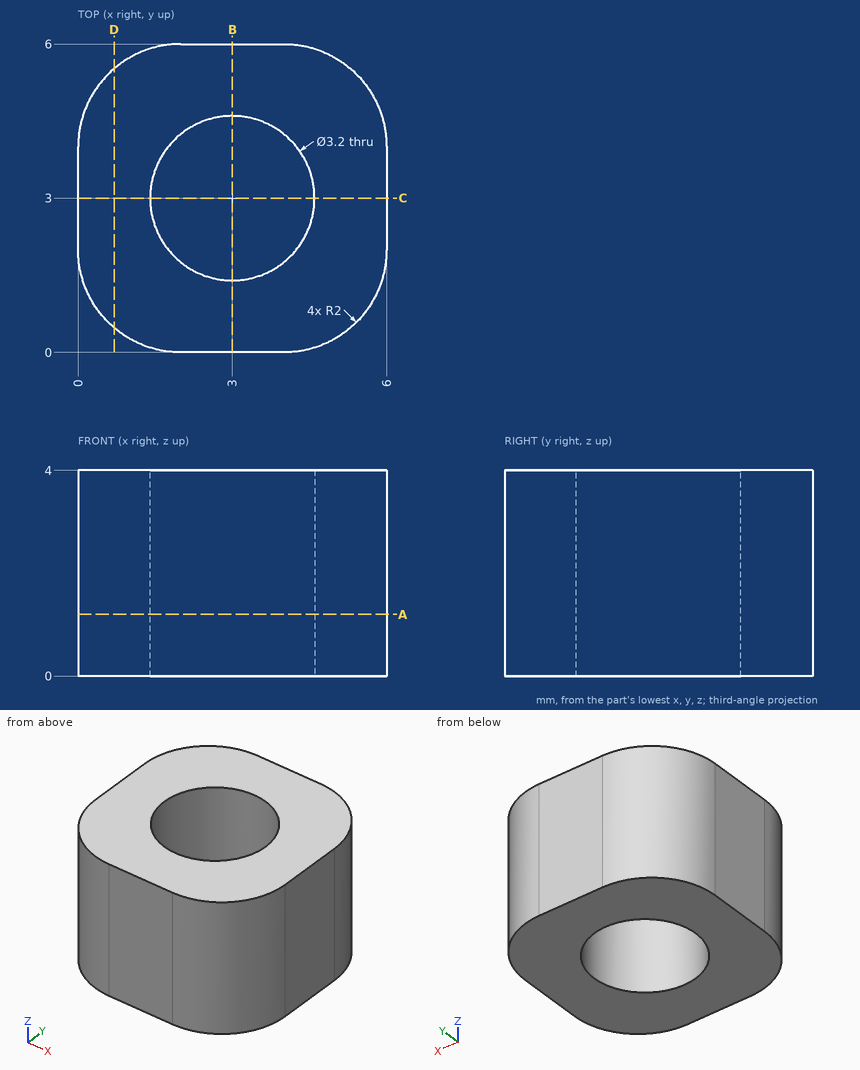
Check sheet for the drawn part. Datum: minimum x, y, z corner. Units: mm. Give positions to 0.01 mm unless a question says otherwise; leave off trailing zeros. Write each loop counter-clockwise with the first axis right and the second up, starting at its lowest first coordinate (ties: lowest second). Pieces come first, ordered by that corner, then holes. Notation, with made-up numbers: M 40.5,-5 L 74.5,-5 A17 cw 74.5,24 Z; hole C 0,-35.75 d10. An arc over 180 degrees is marked long. Write item = value, one per line.
(1) Go/stop test with flat-tipped pins: pin 1 Ø1.5 at (x, z) = (1, 0.5) entering from +Y; pin 2 Ø2 at (y, z) = (5, 2) entering from -X. Record where each tip stops, or that it passes through.
Found:
pin_1 = 5.98
pin_2 = 0
(2) Material ranges on line 1 (Y direction, x = 3, z = 3.1); line 2 (Y direction, x = 3.5, z = 3.65), recorded low to high.
Found:
line_1 = 0 to 1.4, 4.6 to 6
line_2 = 0 to 1.48, 4.52 to 6
(3) Sectioned sample at D-D (x = 0.7). Record the cut outline in (y, z), then the cut area to 3 significant figures.
Found:
outline = M 0.48,0 L 5.52,0 L 5.52,4 L 0.48,4 Z
area = 20.2 mm2
(4) Sectioned sample at B-B (x = 3). Record the cut outline in (y, z).
Found:
outline = M 0,0 L 1.4,0 L 1.4,4 L 0,4 Z; M 4.6,0 L 6,0 L 6,4 L 4.6,4 Z
(5) Sectioned sample at A-A (z = 1.2). Record the cut outline in (x, y), then the cut area to 3 significant figures.
Found:
outline = M 0,2 A2 ccw 2,0 L 4,0 A2 ccw 6,2 L 6,4 A2 ccw 4,6 L 2,6 A2 ccw 0,4 Z; hole C 3,3 d3.2
area = 24.5 mm2
